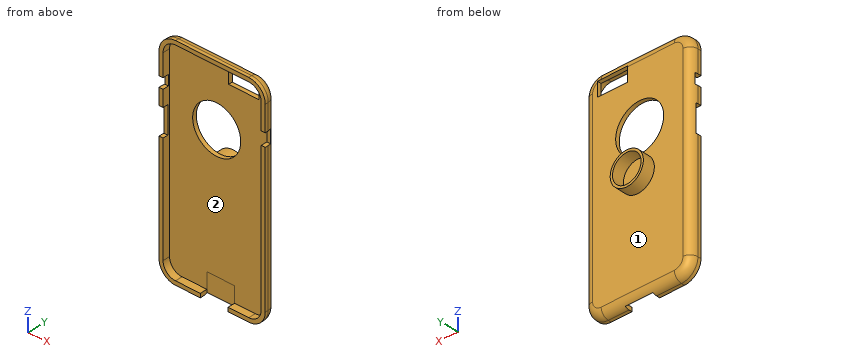
from build123d import *

# Parameters (mm, degrees)
F0_W          = 67.1
F0_H          = 138.6
F1_DEPTH      = 7.1
F2_R          = 10.4245741623
F3_T          = -2.54
F4_W          = 19.2213095725
F4_H          = 9.1803260148
F5_DEPTH      = 12.5
F6_W          = 17.5000010058
F6_H          = 4.661475262
F7_DEPTH      = 12.5
F8_W          = 3.0759498477
F8_H          = 14.1388773918
F9_DEPTH      = 12.5
F10_W         = 3.7169439722
F10_H         = 6.5781623125
F11_DEPTH     = 12.5
F12_W         = 3.3410489097
F12_H         = 17.2911705449
F13_DEPTH     = 12.5
F14_W         = 3.904892784
F14_H         = 8.2696899772
F15_DEPTH     = 12.5
F16_T1_DEPTH  = 117.7508516753
F16_T3_DEPTH  = 46.2508516753
F16_T6_ANGLE  = 90
F16_T8_ANGLE  = 90
F16_T10_ANGLE = 90
F16_T12_ANGLE = 90
F17_R         = 15.1895589548
F18_DEPTH     = 12.5
F19_R         = 10.4830955048
F19_R_2       = 9.0277735867
F20_DEPTH     = 7.7


# Not quite as in the source:
# - a fillet or chamfer that OpenCascade refuses, or shapes differently, is made with other operations: its cross-section is extruded or revolved along the edge and cut away or added


with BuildPart() as f1:
    # F0 (on Front) → F1 (new body)
    with BuildSketch(Plane.XZ):
        Rectangle(F0_W, F0_H)
    extrude(amount=F1_DEPTH)

    # F2
    f2_edges = [f1.edges().sort_by_distance(p)[0] for p in [
        (33.55, -3.55, 69.3),
        (-33.55, -3.55, 69.3),
        (-33.55, -3.55, -69.3),
        (33.55, -3.55, -69.3),
    ]]
    fillet(f2_edges, radius=F2_R)

    # F3
    f3_openings = [f1.faces().sort_by_distance(p)[0] for p in [
        (0, -7.1, 0),
    ]]
    offset(amount=F3_T, openings=f3_openings)

    # F4 (on Front) → F5 (cut, symmetric)
    with BuildSketch(Plane.XZ):
        with Locations((15.9221310169, 60.1024609059)):
            Rectangle(F4_W, F4_H)
    extrude(amount=F5_DEPTH, both=True, mode=Mode.SUBTRACT)

    # F6 (on face) → F7 (cut, symmetric)
    with BuildSketch(Plane(origin=(0, 0, -69.3), x_dir=(1, 0, 0), z_dir=(0, 0, -1))):
        with Locations((1.2909830548, 4.769262369)):
            Rectangle(F6_W, F6_H)
    extrude(amount=F7_DEPTH, both=True, mode=Mode.SUBTRACT)

    # F8 (on Front) → F9 (cut, symmetric)
    with BuildSketch(Plane.XZ):
        with Locations((35.5030968785, 36.7480814457)):
            Rectangle(F8_W, F8_H)
    extrude(amount=F9_DEPTH, both=True, mode=Mode.SUBTRACT)

    # F10 (on face) → F11 (cut, symmetric)
    with BuildSketch(Plane(origin=(-33.55, 0, 0), x_dir=(0, -1, 0), z_dir=(-1, 0, 0))):
        with Locations((5.2415280139, 41.4424240589)):
            Rectangle(F10_W, F10_H)
    extrude(amount=F11_DEPTH, both=True, mode=Mode.SUBTRACT)

    # F12 (on face) → F13 (cut, symmetric)
    with BuildSketch(Plane(origin=(-33.55, 0, 0), x_dir=(0, -1, 0), z_dir=(-1, 0, 0))):
        with Locations((5.4294755451, 19.1706451587)):
            Rectangle(F12_W, F12_H)
    extrude(amount=F13_DEPTH, both=True, mode=Mode.SUBTRACT)

    # F14 (on face) → F15 (cut, symmetric)
    with BuildSketch(Plane.YZ.offset(33.55)):
        with Locations((-5.147553608, 38.5292358696)):
            Rectangle(F14_W, F14_H)
    extrude(amount=F15_DEPTH, both=True, mode=Mode.SUBTRACT)

    # F16: fillet of radius 5 on 1 edges, made by hand

    # F16_s2 → F16_t1 (cut)
    with BuildSketch(Plane.XY.offset(-58.8754258377)):
        with BuildLine():
            ThreePointArc((33.55, -5), (32.0855339059, -1.4644660941), (28.55, 0))
            Line((28.55, 0), (33.55, 0))
            Line((33.55, 0), (33.55, -5))
        make_face()
        with BuildLine():
            ThreePointArc((-28.55, 0), (-32.0855339059, -1.4644660941), (-33.55, -5))
            Line((-33.55, -5), (-33.55, 0))
            Line((-33.55, 0), (-28.55, 0))
        make_face()
    extrude(amount=F16_T1_DEPTH, mode=Mode.SUBTRACT)

    # F16_s4 → F16_t3 (cut)
    with BuildSketch(Plane.YZ.offset(-23.1254258377)):
        with BuildLine():
            ThreePointArc((0, 64.3), (-1.4644660941, 67.8355339059), (-5, 69.3))
            Line((-5, 69.3), (0, 69.3))
            Line((0, 69.3), (0, 64.3))
        make_face()
        with BuildLine():
            ThreePointArc((0, -64.3), (-1.4644660941, -67.8355339059), (-5, -69.3))
            Line((-5, -69.3), (0, -69.3))
            Line((0, -69.3), (0, -64.3))
        make_face()
    extrude(amount=F16_T3_DEPTH, mode=Mode.SUBTRACT)

    # F16_s5 → F16_t6 (revolve, cut)
    with BuildSketch(Plane.XY.offset(-58.8754258377)):
        with BuildLine():
            ThreePointArc((28.55, 0), (32.0855339059, -1.4644660941), (33.55, -5))
            Line((33.55, -5), (33.55, 0))
            Line((33.55, 0), (28.55, 0))
        make_face()
    revolve(axis=Axis((23.1254258377, 0, -58.8754258377), (0, 1, 0)), revolution_arc=F16_T6_ANGLE, mode=Mode.SUBTRACT)

    # F16_s7 → F16_t8 (revolve, cut)
    with BuildSketch(Plane.XY.offset(58.8754258377)):
        with BuildLine():
            ThreePointArc((28.55, 0), (32.0855339059, -1.4644660941), (33.55, -5))
            Line((33.55, -5), (33.55, 0))
            Line((33.55, 0), (28.55, 0))
        make_face()
    revolve(axis=Axis((23.1254258377, 0, 58.8754258377), (0, -1, 0)), revolution_arc=F16_T8_ANGLE, mode=Mode.SUBTRACT)

    # F16_s9 → F16_t10 (revolve, cut)
    with BuildSketch(Plane.YZ.offset(-23.1254258377)):
        with BuildLine():
            ThreePointArc((0, 64.3), (-1.4644660941, 67.8355339059), (-5, 69.3))
            Line((-5, 69.3), (0, 69.3))
            Line((0, 69.3), (0, 64.3))
        make_face()
    revolve(axis=Axis((-23.1254258377, 0, 58.8754258377), (0, -1, 0)), revolution_arc=F16_T10_ANGLE, mode=Mode.SUBTRACT)

    # F16_s11 → F16_t12 (revolve, cut)
    with BuildSketch(Plane.XY.offset(-58.8754258377)):
        with BuildLine():
            ThreePointArc((-28.55, 0), (-32.0855339059, -1.4644660941), (-33.55, -5))
            Line((-33.55, -5), (-33.55, 0))
            Line((-33.55, 0), (-28.55, 0))
        make_face()
    revolve(axis=Axis((-23.1254258377, 0, -58.8754258377), (0, -1, 0)), revolution_arc=F16_T12_ANGLE, mode=Mode.SUBTRACT)

    # F17 (on Front) → F18 (cut, symmetric)
    with BuildSketch(Plane.XZ):
        with Locations((-1.2289978711, 26.4862392154)):
            Circle(F17_R)
    extrude(amount=F18_DEPTH, both=True, mode=Mode.SUBTRACT)

    # F19 (on Front) → F20 (join)
    with BuildSketch(Plane.XZ):
        Circle(F19_R)
        Circle(F19_R_2, mode=Mode.SUBTRACT)
    extrude(amount=-F20_DEPTH)


solid = f1.part
Could you check a few things on this model? Use its own coordinates, in mm. Face numbers are marked on the shaded views. Coordinates: 2 decimals unless noted, no trailing zeros. Loops run counter-clockwise (first coordinate to the right, second up) from the corner with the lowest first, then second, coordinate; pieces in that order, holes last.
1. We'd pull the mould along X, two halves only. Please class the marked faces 1 and 2: released by +X, released by -X, zero draft, split by the parting line, or undercut.
2. Imagine slicing it at A-A (x = 17). Please give me the cut outline in (y, z), and give its area (3 significant figures).
3. Imagine slicing it at D-D (y = 4.5). Please give me the cut outline in (x, z), and give its area (3 significant figures).
4. I need wall thicknesses on L1, parallel to Z at x = 0, y = 5.5; L2, parallel to Z at x = 16.5, y = -5; L3, parallel to X at y = -5, z = -23. Which ranges of each line are inside material? Lowest first, please.
5. For P1, Ø6, axis at x = 9, z = 35.5, coming from the -Y side; P2, Ø1, axis at y = 5, z = 4, coming from the -X side; P3, Ø9, axis at x = 3, z = -4, coming from the +Y side; P4, Ø1.4, axis at y = -3.5, z = -63.5, coming from the -X side, each with a flat end and sliding along its axis, tell me the tip position at first contact or that it passes through.
6. Imagine slicing it at C-C (z = 24). Please give me the cut outline in (x, y), and give its area (3 significant figures).
7. Imagine slicing it at B-B (z = 0). Please give me the cut outline in (x, y).
Computed values:
1. face 1: zero draft
1. face 2: undercut
2. outline: (-7.1, -69.3) - (-5, -69.3) arc R5 ccw to (0, -64.3) - (0, 55.51) - (-2.54, 55.51) - (-2.54, -66.76) - (-7.1, -66.76) - close; (-7.1, 66.76) - (-2.54, 66.76) - (-2.54, 64.69) - (-0.02, 64.69) arc R5 ccw to (-5, 69.3) - (-7.1, 69.3) - close
2. area: 341 mm2
3. outline: circle Ø20.97 at (0, 0); hole circle Ø18.06 at (0, 0)
3. area: 89.2 mm2
4. L1: z = -10.48 to -9.03, 9.03 to 10.48
4. L2: z = -69.3 to -66.76, 66.76 to 69.3
4. L3: x = -33.55 to -31.01, 31.01 to 33.55
5. P1: stops at y = -2.54
5. P2: stops at x = -9.88
5. P3: stops at y = 7.7
5. P4: stops at x = -32.6
6. outline: (-33.39, -3.76) - (-31.01, -3.76) - (-31.01, -2.54) - (-16.21, -2.54) - (-16.21, 0) - (-28.55, 0) arc R5 ccw to start; (13.76, -2.54) - (31.01, -2.54) - (31.01, -7.1) - (33.55, -7.1) - (33.55, -5) arc R5 ccw to (28.55, 0) - (13.76, 0) - close
6. area: 98.3 mm2
7. outline: (-33.55, -7.1) - (-31.01, -7.1) - (-31.01, -2.54) - (31.01, -2.54) - (31.01, -7.1) - (33.55, -7.1) - (33.55, -5) arc R5 ccw to (28.55, 0) - (10.48, 0) - (10.48, 7.7) - (9.03, 7.7) - (9.03, 0) - (-9.03, 0) - (-9.03, 7.7) - (-10.48, 7.7) - (-10.48, 0) - (-28.55, 0) arc R5 ccw to (-33.55, -5) - close
